The model under review builds one solid part; all positions refer to its coordinate system, in mm. A direction names the side the tool comes from. Coordinates: 2 decimals unless noted, no trailing zeros. Answer in a Markdown table with one row per item. Add a question column.
(1) For P1, Ø5.5, axis at x = 105.5, y = -188.5, coming from the +Z side; P2, Ø6.5, axis at x = -105, y = -190, coming from the -Z side, all flat-tipped, find the tip position at first contact; note any pin that passes through.
(2) Machinability: for faces 4 (the flat face through (2, -200, 6)), 5 (the cylindrical face through (-108.72, -185.95, 9.66)), which of the approach directions +Z, -Z, +X, -X, +Y, -Y give a long, thin tool a straight path to every point of the face, cutting with its end or side? Answer none if there is none.
(3) Mouldability with a two-part tool opening along Y and no side actions: class faces 1 (the flat face through (-125, -3, 6)), 2 (the flat face through (-108, 190, 6.7)), 3 (the flat face through (-2, 200, 6)) as +Y half, -Y half, draft (parallel to the pull), parting line (faces both ways), or undercut.
(4) For line 1 along Y through (x, z) = (-105, 11.2); line 2 along X through (y, z) = (190, 2); line 3 along Y through (x, z) = (-105, 5), list the stretches that pass through material, from the lowest coordinate up.
Autodesk Inventor part; units mm, degrees
ref_plane "YZ Plane" through (0, 0, 0) normal (1, 0, 0) x (0, 1, 0)
ref_plane "XZ Plane" through (0, 0, 0) normal (0, 1, 0) x (-1, 0, 0)
ref_plane "XY Plane" through (0, 0, 0) normal (0, 0, 1) x (1, 0, 0)
sketch "Sketch1" plane through (0, 0, 0) normal (0, 0, 1) x (1, 0, 0)
  line L0 (-125, 200) -> (125, 200)
  line L1 (125, 200) -> (125, -200)
  line L2 (125, -200) -> (-125, -200)
  line L3 (-125, -200) -> (-125, 200)
  point P0 (0, 0)
  dimension "d0" = 250
  dimension "d1" = 400
  dimension "d2" = 125
  dimension "d3" = 200
extrude "Extrusion1" add sketch "Sketch1" along normal blind 12.7
sketch "Sketch2" plane through (0, 0, 12.7) normal (0, 0, 1) x (1, 0, 0)
  line L0 (-125, -200) -> (125, -200)
  line L1 (125, -200) -> (125, 200)
  circle A0 centre (105, -190) radius 2.75
  point P0 (0, 0)
  dimension "d6" = 5.5
  dimension "d7" = 10
  dimension "d8" = 20
hole "Hole1" at (105, -190, 12.7) direction (0, 0, -1) diameter 5 end through all counterbore diameter 11 counterbore depth 6
pattern_linear "Rectangular Pattern1" count 2 spacing 210 along (-1, 0, 0) count 2 spacing 380 along (0, 1, 0) of "Hole1"
properties part number "two_part_wastebaord" material "Wood (Walnut)"
Outcome:
| question | item | result |
|---|---|---|
| 1 | P1 | z = 6.7 |
| 1 | P2 | z = 0 |
| 2 | face 4 | +Z, -Z, +X, -X, -Y |
| 2 | face 5 | +Z |
| 3 | face 1 | draft |
| 3 | face 2 | undercut |
| 3 | face 3 | +Y half |
| 4 | line 1 | -200 to -195.5, -184.5 to 184.5, 195.5 to 200 |
| 4 | line 2 | -125 to -107.5, -102.5 to 102.5, 107.5 to 125 |
| 4 | line 3 | -200 to -192.5, -187.5 to 187.5, 192.5 to 200 |
